Work out the finished part from the listing and answer in its coordinate system (mm). A direction names the side the tool comes from. Give positions to 0.01 mm unless a question says otherwise; leave off trailing zeros. Loops run counter-clockwise (first coordinate to the right, second up) from the corner with the lowest first, then second, coordinate; pieces in that order, holes last. Notation, with made-up numbers: M 71.25,40.25 L 107.25,40.25 A29 ccw 107.25,76.25 Z; hole C 31,-3.5 d1. An arc over 180 degrees is marked long. Write item = value, one per line. Start each with the question number.
1. Section C-C on x = -14 is taken. Determine the outline of the cut face in (y, z).
2. Section A-A on z = 57.15 is taken. Determine the outline of the cut face in (x, y).
3. For faces 1 (the face through (0, 44.45, 25)), 2 (the face through (0, 51, 19.05)), 3 (the face through (0, 31, 0)), determine the directions among +Z, -Z, +X, -X, +Y, -Y from which every point of the face is accessible in a straight line to the end or side of a thin tool.
4. Consider L1, parallel to Z at x = 0, y = 61.5; L2, parallel to Y at x = 0, z = 13.25; L3, parallel to X at y = 60, z = 57. Determine where each line is inside the solid, lowest interval first. Write a range as [from, to].
5. The mould has two halves that part along Y. Classify faces 4 (the face through (-0.07, 60.349, 55.564)), 5 (the face through (0.704, 14.166, 5.656)), 6 (the face through (0, 63.5, 31)), 7 (the face through (0, 32, 32)): released by +Y, released by -Y, zero draft, split by the parting line, or undercut.
6. Section D-D on y = 13.5 is taken. Determine the outline of the cut face in (x, z).
7. Flat-ended cylindrical pins translate along their axes: pin 1 Ø4 at (x, y) = (0.1, 12.7) entering from +Z; pin 2 Ø1 at (x, y) = (-12, 17) entering from +Z; pin 3 Ø6 at (x, y) = (6, 20) entering from +Z. Find the tip coordinate at first contact, or state that the pin passes through.
Autodesk Fusion 360 part; units mm, degrees
sketch "Sketch1" plane through (0, 0, 0) normal (1, 0, 0) x (0, 1, 0)
  line L0 (0, 0) -> (63.5, 0)
  line L1 (63.5, 0) -> (63.5, 63.5)
  line L2 (63.5, 63.5) -> (0, 0)
  dimension "d1" = 63.5
extrude "Extrude1" add sketch "Sketch1" along normal mid plane 38.1
sketch "Sketch2" plane through (0, 0, 0) normal (0, 0, -1) x (1, 0, 0)
  line L0 (-19.05, -63.5) -> (19.05, -63.5)
  line L1 (19.05, -63.5) -> (19.05, 0)
  line L2 (19.05, 0) -> (-19.05, 0)
  line L3 (-19.05, 0) -> (-19.05, -63.5)
  circle A0 centre (0.0962, -12.6996) radius 6.8134
  circle A1 centre (0, -50.8) radius 6.965
  dimension "d10" = 12.7
  dimension "d11" = 12.7
sketch "Sketch3" plane through (0, 63.5, 0) normal (0, 1, 0) x (-1, 0, 0)
  line L0 (19.05, 63.5) -> (-19.05, 63.5)
  line L1 (-19.05, 63.5) -> (-19.05, 0)
  line L2 (-19.05, 0) -> (19.05, 0)
  line L3 (19.05, 0) -> (19.05, 63.5)
  circle A0 centre (0.3187, 25.398) radius 3.175
  circle A1 centre (0, 57.15) radius 3.175
  dimension "d12" = 25.4
  dimension "d13" = 6.35
  dimension "d14" = 6.35
  dimension "d15" = 6.35
hole "Hole3" at (0, 63.5, 57.15) at (-0.3187, 63.5, 25.398) direction (0, -1, 0) diameter 3.175 depth 19.05 tip angle 180
hole "Hole4" at (0, 50.8, 0) at (0.0962, 12.6996, 0) direction (0, 0, 1) diameter 3.175 depth 19.05 tip angle 180
equation "d17 = ( 1 / 8 ) * 1 in"
Verdict:
q1.outline = M 0,0 L 63.5,0 L 63.5,63.5 Z
q2.outline = M -19.05,57.15 L -1.59,57.15 L -1.59,63.5 L -19.05,63.5 Z; M 1.59,57.15 L 19.05,57.15 L 19.05,63.5 L 1.59,63.5 Z
q3.face_1 = +Y
q3.face_2 = -Z
q3.face_3 = -Z, +X, -X, +Y, -Y
q4.L1 = [0, 23.84], [26.95, 55.56], [58.74, 61.5]
q4.L2 = [14.28, 49.21], [52.39, 63.5]
q4.L3 = [-19.05, -1.58], [1.58, 19.05]
q5.face_4 = zero draft
q5.face_5 = undercut
q5.face_6 = released by +Y
q5.face_7 = released by -Y
q6.outline = M -19.05,0 L -1.27,0 L -1.27,13.5 L -19.05,13.5 Z; M 1.47,0 L 19.05,0 L 19.05,13.5 L 1.47,13.5 Z
q7.pin_1 = 14.7
q7.pin_2 = 17.5
q7.pin_3 = 23
